from build123d import *

# Parameters (mm, degrees)
BASEPLATE_DEPTH = 8
SKETCH_4_R      = 12
PIVOTA_DEPTH    = 20
SKETCH_5_R      = 12
PIVOTD_DEPTH    = 20


with BuildPart() as part:
    # 草图3 → BasePlate (new body)
    with BuildSketch(Plane.XY):
        with BuildLine():
            Line((85, 0), (195, 0))
            ThreePointArc((195, 0), (198.535533906, 1.464466094), (200, 5))
            Line((200, 5), (200, 25))
            ThreePointArc((200, 25), (198.535533906, 28.535533906), (195, 30))
            Line((195, 30), (85, 30))
            ThreePointArc((85, 30), (81.464466094, 28.535533906), (80, 25))
            Line((80, 25), (80, 5))
            ThreePointArc((80, 5), (81.464466094, 1.464466094), (85, 0))
        make_face()
    extrude(amount=BASEPLATE_DEPTH)

    # 草图4 → PivotA (add)
    with BuildSketch(Plane.XY):
        with Locations(Location((100, 12, 0), (0, 0, 270))):
            Circle(SKETCH_4_R)
    extrude(amount=PIVOTA_DEPTH)

    # 草图5 → PivotD (add)
    with BuildSketch(Plane.XY):
        with Locations(Location((180, 12, 0), (0, 0, 270))):
            Circle(SKETCH_5_R)
    extrude(amount=PIVOTD_DEPTH)


solid = part.part
Input: part model. Units: mm. Frame: model coordinates. A direction names the side the tool comes from. Coordinates: 2 decimals unless noted, no trailing zeros. Loops run counter-clockwise (first coordinate to the right, second up) from the corner with the lowest first, then second, coordinate; pieces in that order, holes last. Notation, with made-up numbers: (-34, 58) -> (-7, 58) arc R6 cw to (-7, 64) -> close; hole circle Ø6 at (-35.5, 40.5). An arc over 180 degrees is marked (long way). One line per item, written item: value.
(1) Cut plane B-B (z = 17.5). Output: boundary loops of the cut face in (x, y).
Answer below:
outline: circle Ø24 at (100, 12); circle Ø24 at (180, 12)
(2) Ray query, line 1 along Z through (x, y) = (122.5, 9); line 2 along X through (y, z) = (22.75, 15.75); line 3 along X through (y, z) = (22, 13.5). Return the intervals inside material, ascending.
Answer below:
line 1: z = 0 to 8
line 2: x = 94.67 to 105.33, 174.67 to 185.33
line 3: x = 93.37 to 106.63, 173.37 to 186.63
(3) Cut plane A-A (y = 12). Output: boundary loops of the cut face in (x, z).
Answer below:
outline: (80, 0) -> (200, 0) -> (200, 8) -> (192, 8) -> (192, 20) -> (168, 20) -> (168, 8) -> (112, 8) -> (112, 20) -> (88, 20) -> (88, 8) -> (80, 8) -> close
(4) Pin query (flat end, axial travel): pin 1 Ø3 at (y, z) = (27, 17) entering from -X; pin 2 Ø4 at (x, y) = (151, 6.5) entering from +Z. Return the tip coordinate at first contact, or that it passes through.
Answer below:
pin 1: passes through
pin 2: stops at z = 8
(5) Draft query along X for faces 1 (the face through (139, 0, 4)), 2 (the face through (81, 2, 4)), 3 (the face through (191.9, 13.56, 13.92)). Return one class per face: pulls with the +X half, pulls with the -X half, needs draft (parallel to the pull), parting line crosses it, or undercut.
Answer below:
face 1: needs draft
face 2: pulls with the -X half
face 3: undercut
(6) Set-up query: faces 4 (the face through (199, 28, 4)), 5 (the face through (108.11, 20.844, 13.916)). Return all of +Z, -Z, +X, -X, +Y, -Y with unobstructed straight access to the full face (end or side cutting, diameter ignored); none if empty.
Answer below:
face 4: +Z, -Z, +X, +Y
face 5: +Z
(7) Cut plane C-C (x = 98). Output: boundary loops of the cut face in (y, z).
Answer below:
outline: (0, 0) -> (30, 0) -> (30, 8) -> (23.83, 8) -> (23.83, 20) -> (0.17, 20) -> (0.17, 8) -> (0, 8) -> close
(8) Cut plane D-D (y = 17.5). Output: boundary loops of the cut face in (x, z).
Answer below:
outline: (80, 0) -> (200, 0) -> (200, 8) -> (190.67, 8) -> (190.67, 20) -> (169.33, 20) -> (169.33, 8) -> (110.67, 8) -> (110.67, 20) -> (89.33, 20) -> (89.33, 8) -> (80, 8) -> close
